Build history of the part. All positions in model axes, mm. Give positions to 0.01 mm unless a question says otherwise; leave off trailing zeros. Write each loop counter-clockwise with the first axis right and the second up, starting at its lowest first coordinate (ties: lowest second). Pieces come first, ordered by that corner, then holes. Notation, with made-up numbers: (63.25, -39.75) -> (107.25, -39.75) arc R13 ccw to (107.25, -22.75) -> close; hole circle Ø2 at (60.5, 80). An arc over 180 degrees is marked (long way). Write item = value, one per line. Start each with the question number.
Q1. Drop a flat-ended pin along its axis: P1, Ø4.5, axis at x = 47.5, z = 0, coming from the +Y side. Give the stop position or say it passes through.
Q2. Mould opens along Z. For faces 1 (the face through (-45.06, 1.1, -0.54)), 2 (the face through (-1, 3.175, 0)), 3 (the face through (49.94, 1.1, -0.54)), 4 (the face through (-1, 2, 5)) say: pulls with the +Z half, pulls with the -Z half, needs draft (parallel to the pull), parting line crosses it, or undercut.
Q3. Saw through at C-C, the plane y = 0.55. List the corners of the cut face in (x, z).
Q4. Wall check: line 1 (X direction, y = 0.55, z = 0); line 2 (Z direction, x = -47.5, y = 1.45); line 3 (X direction, y = 3.05, z = 0.5). Give the ranges that are in metal, low to high.
Q5. Saw through at A-A, the plane z = 0. List the corners of the cut face in (x, y) (3 decimals).
Q6. Saw through at B-B, the plane x = -47.5. List the corners of the cut face in (y, z) (3 decimals).
from build123d import *

# Parameters (mm, degrees)
SKETCH1_W                      = 105
SKETCH1_H                      = 10
BOSS_EXTRUDE1_DEPTH            = 3.175
M6X1_0_TAPPED_HOLE1_AT_2_COUNT = 2
M6X1_0_TAPPED_HOLE1_AT_2_PITCH = 95


with BuildPart() as part:
    # Sketch1 → Boss-Extrude1 (new body)
    with BuildSketch(Plane(origin=(0, 0, 0), x_dir=(1, 0, 0), z_dir=(0, 1, 0))):
        Rectangle(SKETCH1_W, SKETCH1_H)
    extrude(amount=BOSS_EXTRUDE1_DEPTH)

    # Sketch4 → M6x1.0 Tapped Hole1 (revolve, cut)
    with BuildSketch(Plane(origin=(47.5, 3.175, 0), x_dir=(0, 0, 1), z_dir=(1, 0, 0))):
        Polygon((0, 0), (0, 3.175), (2.5, 3.175), (2.5, 1), (3.5, 0), align=None)
    m6x1_0_tapped_hole1 = revolve(axis=Axis((47.5, 9.525, 0), (0, -1, 0)), mode=Mode.SUBTRACT)

    # M6x1.0 Tapped Hole1 at 2: M6x1.0 Tapped Hole1 ×2
    with Locations(*[(-i * M6X1_0_TAPPED_HOLE1_AT_2_PITCH, 0, 0) for i in range(1, M6X1_0_TAPPED_HOLE1_AT_2_COUNT)]):
        add(m6x1_0_tapped_hole1, mode=Mode.SUBTRACT)


solid = part.part
Report:
q1.P1 = through
q2.face_1 = undercut
q2.face_2 = needs draft
q2.face_3 = undercut
q2.face_4 = pulls with the +Z half
q3.outline = (-52.5, -5) -> (52.5, -5) -> (52.5, 5) -> (-52.5, 5) -> close; hole circle Ø5 at (-47.5, 0); hole circle Ø5 at (47.5, 0)
q4.line_1 = -52.5 to -50, -45 to 45, 50 to 52.5
q4.line_2 = -5 to -2.5, 2.5 to 5
q4.line_3 = -52.5 to -50.84, -44.16 to 44.16, 50.84 to 52.5
q5.outline = (-52.5, 0) -> (-50, 0) -> (-50, 2.175) -> (-51, 3.175) -> (-52.5, 3.175) -> close; (-45, 0) -> (45, 0) -> (45, 2.175) -> (44, 3.175) -> (-44, 3.175) -> (-45, 2.175) -> close; (50, 0) -> (52.5, 0) -> (52.5, 3.175) -> (51, 3.175) -> (50, 2.175) -> close
q6.outline = (0, -5) -> (3.175, -5) -> (3.175, -3.5) -> (2.175, -2.5) -> (0, -2.5) -> close; (0, 2.5) -> (2.175, 2.5) -> (3.175, 3.5) -> (3.175, 5) -> (0, 5) -> close
